Geometry: see drawing. Coordinates: mm, zero at the bounding-box minimum. A direction names the side the tool comes from. Coordinates: 2 decimals unless noted, no trailing zeros. Write each loop counter-clockwise with the first axis right and the second up, starting at its lowest first coordinate (ties: lowest second). Pieces come first, ordered by that corner, then holes.
1) Set-up query: the marked faces 1 and 2. Return all of +Z, -Z, +X, -X, +Y, -Y with unobstructed straight access to the full face (end or side cutting, diameter ignored); none if empty.
2) Section query A-A (y = 9.3). Output: boundary loops of the cut face in (x, z).
3) Section query C-C (z = 9). Output: boundary loops of the cut face in (x, y).
4) Line query: L1, parallel to Y at x = 9.25, z = 56; L2, parallel to X at y = 1.25, z = 29; L3, parallel to Z at x = 12.25, y = 8.25. Output: solid intervals per line, ascending.
5) Draft query along Y for the marked faces 3, 4, 5 and 6. Return one class per face: pulls with the +Y half, pulls with the -Y half, needs draft (parallel to the pull), parting line crosses it, or undercut.
6) Section query B-B (x = 6.5). Output: boundary loops of the cut face in (y, z).
7) Pin query (flat end, axial travel): pin 1 Ø2 at (x, y) = (2.5, 6) entering from -Z; pin 2 Ø10 at (y, z) = (22, 35.5) entering from -X. Return the tip coordinate at first contact, or that it passes through.
8) Section query D-D (z = 36). Output: boundary loops of the cut face in (x, y).
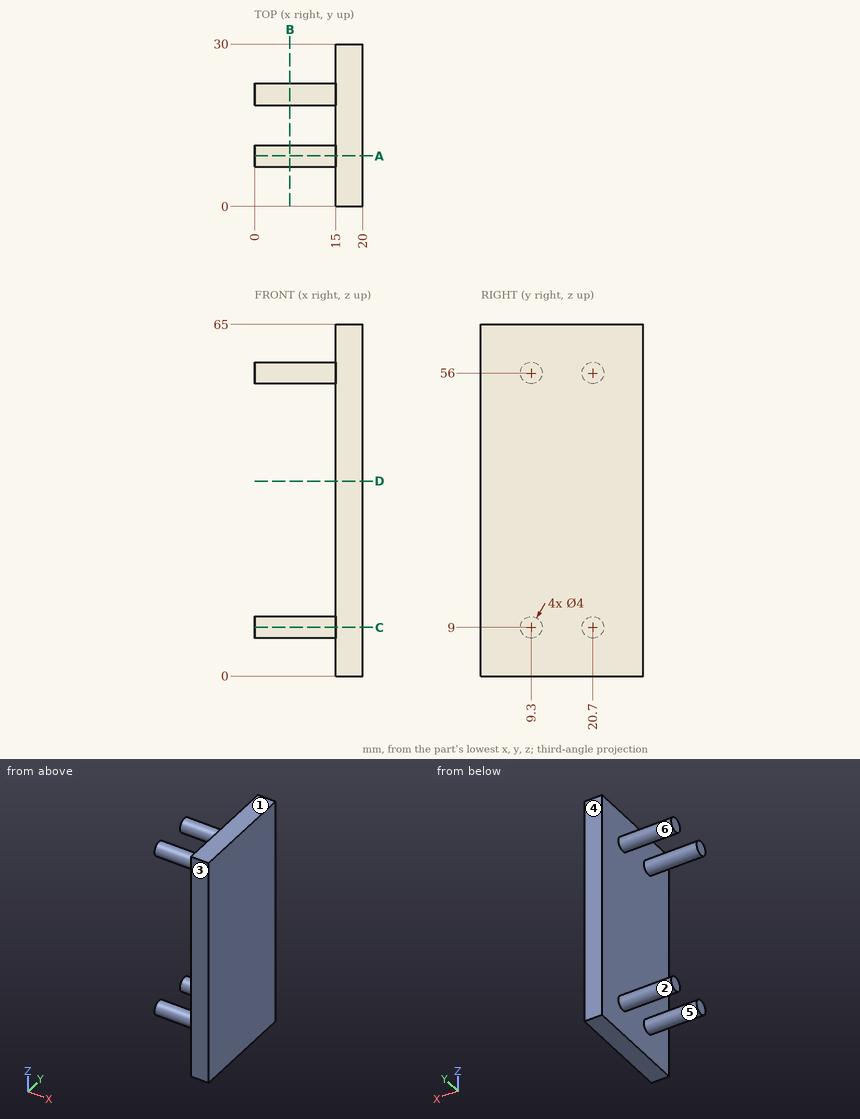
Answer:
1. face 1: +Z, +X, -X, +Y, -Y
1. face 2: -X
2. outline: (0, 7) - (15, 7) - (15, 0) - (20, 0) - (20, 65) - (15, 65) - (15, 58) - (0, 58) - (0, 54) - (15, 54) - (15, 11) - (0, 11) - close
3. outline: (0, 7.3) - (15, 7.3) - (15, 0) - (20, 0) - (20, 30) - (15, 30) - (15, 22.7) - (0, 22.7) - (0, 18.7) - (15, 18.7) - (15, 11.3) - (0, 11.3) - close
4. L1: y = 7.3 to 11.3, 18.7 to 22.7
4. L2: x = 15 to 20
4. L3: z = 7.3 to 10.7, 54.3 to 57.7
5. face 3: pulls with the -Y half
5. face 4: pulls with the +Y half
5. face 5: undercut
5. face 6: undercut
6. outline: circle Ø4 at (9.3, 9); circle Ø4 at (9.3, 56); circle Ø4 at (20.7, 9); circle Ø4 at (20.7, 56)
7. pin 1: passes through
7. pin 2: stops at x = 15
8. outline: (15, 0) - (20, 0) - (20, 30) - (15, 30) - close
